```python
from build123d import *

# Parameters (mm, degrees)
F0_W     = 7.5
F0_H     = 7.5
F1_DEPTH = 25
F2_R     = 5
F3_DEPTH = 25.001


with BuildPart() as f1:
    # F0 (on Top) → F1 (new body)
    with BuildSketch(Plane.XY):
        with BuildLine():
            Line((20, 6.5), (20, 20))
            Line((20, 20), (6.5, 20))
            Line((6.5, 20), (6.5, 16.5))
            Line((6.5, 16.5), (10.5, 16.5))
            Line((10.5, 16.5), (10.5, 11.914214))
            Line((10.5, 11.914214), (4.905379, 6.319593))
            ThreePointArc((4.905379, 6.319593), (2.59261, 7.568248), (0, 8))
            ThreePointArc((0, 8), (-2.59261, 7.568248), (-4.905379, 6.319593))
            Line((-4.905379, 6.319593), (-10.5, 11.914214))
            Line((-10.5, 11.914214), (-10.5, 16.5))
            Line((-10.5, 16.5), (-6.5, 16.5))
            Line((-6.5, 16.5), (-6.5, 20))
            Line((-6.5, 20), (-20, 20))
            Line((-20, 20), (-20, 6.5))
            Line((-20, 6.5), (-16.5, 6.5))
            Line((-16.5, 6.5), (-16.5, 10.5))
            Line((-16.5, 10.5), (-11.914214, 10.5))
            Line((-11.914214, 10.5), (-6.319593, 4.905379))
            ThreePointArc((-6.319593, 4.905379), (-7.568248, 2.59261), (-8, 0))
            ThreePointArc((-8, 0), (-7.568248, -2.59261), (-6.319593, -4.905379))
            Line((-6.319593, -4.905379), (-11.914214, -10.5))
            Line((-11.914214, -10.5), (-16.5, -10.5))
            Line((-16.5, -10.5), (-16.5, -6.5))
            Line((-16.5, -6.5), (-20, -6.5))
            Line((-20, -6.5), (-20, -20))
            Line((-20, -20), (20, -20))
            Line((20, -20), (20, -6.5))
            Line((20, -6.5), (16.5, -6.5))
            Line((16.5, -6.5), (16.5, -10.5))
            Line((16.5, -10.5), (11.914214, -10.5))
            Line((11.914214, -10.5), (6.319593, -4.905379))
            ThreePointArc((6.319593, -4.905379), (7.568248, -2.59261), (8, 0))
            ThreePointArc((8, 0), (7.568248, 2.59261), (6.319593, 4.905379))
            Line((6.319593, 4.905379), (11.914214, 10.5))
            Line((11.914214, 10.5), (16.5, 10.5))
            Line((16.5, 10.5), (16.5, 6.5))
            Line((16.5, 6.5), (20, 6.5))
        make_face()
        with Locations((-15.25, -15.25)):
            Rectangle(F0_W, F0_H, mode=Mode.SUBTRACT)
        with BuildLine():
            Line((4.905379, -6.319593), (10.5, -11.914214))
            Line((10.5, -11.914214), (10.5, -19))
            Line((10.5, -19), (-10.5, -19))
            Line((-10.5, -19), (-10.5, -11.914214))
            Line((-10.5, -11.914214), (-4.905379, -6.319593))
            ThreePointArc((-4.905379, -6.319593), (-2.59261, -7.568248), (0, -8))
            ThreePointArc((0, -8), (2.59261, -7.568248), (4.905379, -6.319593))
        make_face(mode=Mode.SUBTRACT)
        with Locations((15.25, -15.25)):
            Rectangle(F0_W, F0_H, mode=Mode.SUBTRACT)
        with Locations((-15.25, 15.25)):
            Rectangle(F0_W, F0_H, mode=Mode.SUBTRACT)
        with Locations((15.25, 15.25)):
            Rectangle(F0_W, F0_H, mode=Mode.SUBTRACT)
    extrude(amount=F1_DEPTH)

    # F2 (on face) → F3 (cut, through all)
    with BuildSketch(Plane.XY.offset(25)):
        Circle(F2_R)
    extrude(amount=-F3_DEPTH, mode=Mode.SUBTRACT)


solid = f1.part
```
Geometry check sheet. Reference: the model listing, model coordinates, mm. A direction names the side the tool comes from. Give positions to 0.01 mm unless a question says otherwise; leave off trailing zeros. Order: outer loops, then holes, each group sorted by start corner. A loop starts at its lowest first (then second) coordinate and runs counter-clockwise, first axis right, second up. Notation, with made-up numbers: (36, 64) - (85, 64) arc R11 ccw to (85, 72) - close; hole circle Ø6 at (-21.75, -39.75). An arc over 180 degrees is marked (long way). Answer in a Markdown table with one row per item. Add a question column.
Q1. Cross-section at D-D, the plane y = -1.5. Enter the section's corners in (x, z).
Q2. Cross-section at A-A, the plane x = 12.5. Enter the section's corners in (y, z), then the cut area to 3 significant figures.
Q3. Material ranges on probe 1 along Y at (x, z) = (-13.5, 18); probe 2 along Y at (x, z) = (-1.5, 1.5); probe 3 along X at (y, z) = (-9, 21.25), recorded low to high. Write a range as from..to.
Q4. Tool access check on faces 4 (the flat face through (18, 6.5, 12)), 5 (the flat face through (9.078, 7.664, 12.325)), 6 (the flat face through (0, 6, 0)). Record the directions out of +Z, -Z, +X, -X, +Y, -Y that give a thin tool (end or side, any length) a straight path to the whole face; none if there is none.
Q5. Gauge pin test, flat end, axial feed: pin 1 (2 mm diameter, centred on y = 1.5, z = 7, fed in from -X). Record the tip position at first contact, or that the pin passes through.
Q6. Cross-section at C-C, the plane x = 1. Enter the section's corners in (y, z), then the cut area to 3 significant figures.
Q7. Mould release check, pull along X, two halves, no side actions. Record for faces 1 (the flat face through (-10.5, 14, 12)), 2 (the flat face through (18, -6.5, 12)), 3 (the flat face through (-20, -13, 12)): pulls with the +X half, pulls with the -X half, needs draft (parallel to the pull), parting line crosses it, or undercut.
Check values:
| question | item | result |
|---|---|---|
| 1 | outline | (-7.86, 0) - (-4.77, 0) - (-4.77, 25) - (-7.86, 25) - close; (4.77, 0) - (7.86, 0) - (7.86, 25) - (4.77, 25) - close |
| 2 | outline | (-20, 0) - (-19, 0) - (-19, 25) - (-20, 25) - close; (-11.5, 0) - (-10.5, 0) - (-10.5, 25) - (-11.5, 25) - close; (10.5, 0) - (11.5, 0) - (11.5, 25) - (10.5, 25) - close; (19, 0) - (20, 0) - (20, 25) - (19, 25) - close |
| 2 | area | 100 mm^2 |
| 3 | probe 1 | y = -20..-19, -11.5..-10.5, 10.5..11.5, 19..20 |
| 3 | probe 2 | y = -20..-19, -7.86..-4.77, 4.77..7.86 |
| 3 | probe 3 | x = -20..-16.5, -10.41..-7.59, 7.59..10.41, 16.5..20 |
| 4 | face 4 | +Z, -Z, +X |
| 4 | face 5 | +Z, -Z |
| 4 | face 6 | -Z, +X, -X, +Y, -Y |
| 5 | pin 1 | stops at x = -7.98 |
| 6 | outline | (-20, 0) - (-19, 0) - (-19, 25) - (-20, 25) - close; (-7.94, 0) - (-4.9, 0) - (-4.9, 25) - (-7.94, 25) - close; (4.9, 0) - (7.94, 0) - (7.94, 25) - (4.9, 25) - close |
| 6 | area | 177 mm^2 |
| 7 | face 1 | undercut |
| 7 | face 2 | needs draft |
| 7 | face 3 | pulls with the -X half |
